Geometry check sheet. Reference: the model listing, model coordinates, mm. A direction names the side the tool comes from. Round coordinates to 2 decimals unless told otherwise and drop trailing zeros. Order: outer loops, then holes, each group sorted by start corner. A loop starts at its lowest first (then second) coordinate and runs counter-clockwise, first axis right, second up.
Solid Edge part; units mm, degrees
sketch "Sketch1" plane through (0, 0, 0) normal (0, -1, 0) x (1, 0, 0)
  line L0 (47.7222, 4.2678) -> (-1.7678, 4.2678)
  line L1 (-1.7678, 4.2678) -> (0, 2.5)
  line L2 (49.49, 2.5) -> (0, 2.5)
  line L3 (49.49, 2.5) -> (47.7222, 4.2678)
extrude "Protrusion1" add sketch "Sketch1" against normal blind 15
sketch "Sketch2" plane through (22.9772, 7.5, 4.2678) normal (0, 0, 1) x (1, 0, 0)
  line L0 (-24.745, 5.5) -> (-24.745, 6.5)
  line L1 (-24.745, 6.5) -> (24.745, 6.5)
  line L2 (24.745, 6.5) -> (24.745, 5.5)
  line L3 (24.745, 5.5) -> (-24.745, 5.5)
extrude "Vyříznutí_1" cut sketch "Sketch2" against normal blind 1.25
sketch "Sketch3" plane through (47.7222, 13.5, 3.6428) normal (-1, 0, 0) x (0, 0, 1)
  line L0 (-0.625, 0.5) -> (0.625, 0.5)
  line L1 (0.625, 0.5) -> (0.625, -0.5)
  line L2 (0.625, -0.5) -> (-0.625, -0.5)
  line L3 (-0.625, -0.5) -> (-0.625, 0.5)
extrude "Vyříznutí_2" cut sketch "Sketch3" against normal blind 7.0597
sketch "Sketch4" plane through (0, 0, 0) normal (-1, 0, 0) x (0, -1, 0)
  line L0 (2.5, 3.9615) -> (0, 3.9615)
  line L1 (0, 3.9615) -> (0, 3.2071)
  line L2 (0, 3.2071) -> (3, 3.2071)
  line L3 (3, 3.2071) -> (3, 4.7071)
  line L4 (3, 4.7071) -> (2.5, 4.7071)
  line L5 (2.5, 4.7071) -> (2.5, 3.9615)
extrude "Vysunutí_2" add sketch "Sketch4" against normal blind 49.49
sketch "Sketch5" plane through (0, 0, 0) normal (-1, 0, 0) x (0, -1, 0)
  line L0 (2.5, 3.9615) -> (0, 3.9615)
  line L1 (0, 3.9615) -> (0, 3.2071)
  line L2 (0, 3.2071) -> (3, 3.2071)
  line L3 (3, 3.2071) -> (3, 4.7071)
  line L4 (3, 4.7071) -> (2.5, 4.7071)
  line L5 (2.5, 4.7071) -> (2.5, 3.9615)
extrude "Protrusion2" add sketch "Sketch5" along normal up to vertex (1.7678 mm away)
sketch "Sketch6" plane through (-0.8839, 7.5, 3.3839) normal (-0.7071, 0, -0.7071) x (0, -1, 0)
  line L0 (10.5, 2.29) -> (10, 2.29)
  line L1 (10, 2.29) -> (10, 0.5)
  line L2 (10, 0.5) -> (7.5, 0.5)
  line L3 (7.5, -0.25) -> (7.5, 0.5)
  line L4 (7.5, -0.25) -> (10.5, -0.25)
  line L5 (10.5, -0.25) -> (10.5, 2.29)
extrude "Vyříznutí_3" cut sketch "Sketch6" along normal blind 2.1617
sketch "Sketch7" plane through (23.8611, 15, 3.3839) normal (0, 1, 0) x (1, 0, 0)
  line L0 (-25.7842, 0.8839) -> (-25.6289, -0.8839)
  line L1 (-25.6289, -0.8839) -> (-23.8611, 0.8839)
  line L2 (-23.8611, 0.8839) -> (-25.7842, 0.8839)
  line L3 (23.8611, -1.3232) -> (25.6289, -1.3232)
  line L4 (25.6289, -1.3232) -> (25.6289, 0.8839)
  line L5 (25.6289, 0.8839) -> (23.8611, -0.8839)
  line L6 (23.8611, -0.8839) -> (23.8611, -1.3232)
extrude "Vyříznutí_5" cut sketch "Sketch7" against normal blind 20.1859
(1) Sectioned sample at C-C, the plane y = 3.25. Record the cut outline in (x, z).
Returned:
outline: (-1.77, 4.27) - (0, 2.5) - (49.49, 2.5) - (47.72, 4.27) - close
(2) Set-up check for faces 5 (the flat face through (24, -1, 3.207)), 6 (the flat face through (48.62, 5.87, 3.37)), 7 (the flat face through (24, 13, 4)), 8 (the flat face through (-0.9, 5.9, 3.4)), 9 (the flat face through (23, 6, 4.268)): record each of +Z, -Z, +X, -X, +Y, -Y from which the full face is reachable in a straight line by a thin tool's end or side.
Returned:
face 5: -Z, +X, -X, -Y
face 6: +Z, +X, +Y, -Y
face 7: +Z, +X, -X
face 8: -Z, -X, +Y, -Y
face 9: +Z, +X, -X, +Y
(3) Draft check along Y on faces 1 (the flat face through (23.3, 14.5, 4.268)), 2 (the flat face through (23, -1, 3.962)), 3 (the flat face through (24, 15, 3)), 4 (the flat face through (23, 14, 4)). Enter one of: released by +Y, released by -Y, zero draft, split by the parting line, or undercut.
Returned:
face 1: zero draft
face 2: undercut
face 3: released by +Y
face 4: undercut
(4) Material ranges on line 1 (Y direction, x = 39, z = 3.9); line 2 (Z direction, x = 14.5, y = 8); line 3 (Z direction, x = 31.5, y = -1.5), recorded low to high.
Returned:
line 1: y = -3 to 13, 14 to 15
line 2: z = 2.5 to 4.27
line 3: z = 3.21 to 3.96
(5) Sectioned sample at B-B, the plane y = -1. Record the cut outline in (x, z), and give its area (3 significant figures).
Returned:
outline: (-1.46, 3.96) - (-0.71, 3.21) - (48.78, 3.21) - (48.03, 3.96) - close
area: 37.3 mm2
(6) Sectioned sample at A-A, the plane x = 4. Record the cut outline in (y, z), and give its area (3 significant figures).
Returned:
outline: (-3, 3.21) - (0, 3.21) - (0, 2.5) - (15, 2.5) - (15, 4.27) - (14, 4.27) - (14, 3.02) - (13, 3.02) - (13, 4.27) - (0, 4.27) - (0, 3.96) - (-2.5, 3.96) - (-2.5, 4.71) - (-3, 4.71) - close
area: 27.9 mm2
(7) Depth check by flat-ended pin: P1, Ø2, axis at x = 15, y = -2, coming from the +Z side; P2, Ø0.9, axis at x = 15.5, y = -2, coming from the -Z side; P3, Ø0.8, axis at x = 27.5, y = 14.5, coming from the +Z side. Enter the tip coordinate at first touch or a pass-through.
Returned:
P1: stops at z = 4.71
P2: stops at z = 3.21
P3: stops at z = 4.27
